For this review, take the finished solid that the model builds, in its own axes (mm). Face numbers are marked on the shaded views. A direction names the side the tool comes from. Coordinates: 2 decimals unless noted, no trailing zeros. Loops run counter-clockwise (first coordinate to the right, second up) from the corner with the lowest first, then second, coordinate; pieces in that order, holes last. Notation, with made-up numbers: M -31.5,38 L -7.5,38 A26 cw -7.5,57 Z; hole C 58.5,-35.5 d9. An arc over 180 degrees is marked long. Use one line per item in the form item = value.
```python
from build123d import *

# Parameters (mm, degrees)
SKETCH_1_W          = 45
SKETCH_1_H          = 45
EXTRUDE_1_DEPTH     = 9.8
SKETCH_2_W          = 4.7
SKETCH_2_H          = 45
EXTRUDE_2_DEPTH     = 45.7
CUT_EXTRUDE_START   = -33.6
CUT_EXTRUDE_2_DEPTH = 33.6
SKETCH_4_R          = 4
CUT_EXTRUDE_3_DEPTH = 72.630929074
SKETCH_6_R          = 6.1
CUT_EXTRUDE_5_DEPTH = 56.686533381
SKETCH_7_W          = 8.2
SKETCH_7_H          = 1
EXTRUDE_3_DEPTH     = 2
SKETCH_8_R          = 10
CUT_EXTRUDE_6_DEPTH = 4.8


# Read off the part's stored shape, not the designer's step: 切除-拉伸2
with BuildPart() as part:
    # 草图1 → 凸台-拉伸1 (new body)
    with BuildSketch(Plane.XY):
        Rectangle(SKETCH_1_W, SKETCH_1_H)
    extrude(amount=EXTRUDE_1_DEPTH)

    # 草图2 → 凸台-拉伸2 (add)
    with BuildSketch(Plane.XY.offset(9.8)):
        with Locations((-14.45, 0)):
            Rectangle(SKETCH_2_W, SKETCH_2_H)
        with Locations((14.45, 0)):
            Rectangle(SKETCH_2_W, SKETCH_2_H)
    extrude(amount=EXTRUDE_2_DEPTH)

    # 切除-拉伸2 outline → 切除-拉伸2 (cut)
    with BuildSketch(Plane.ZY.offset(16.8).offset(CUT_EXTRUDE_START)):
        with BuildLine():
            Line((55.5, 22.5), (33, 22.5))
            ThreePointArc((33, 22.5), (48.909902577, 15.909902577), (55.5, 0))
            Line((55.5, 0), (55.5, 22.5))
        make_face()
        with BuildLine():
            Line((55.5, -22.5), (55.5, 0))
            ThreePointArc((55.5, 0), (48.909902577, -15.909902577), (33, -22.5))
            Line((33, -22.5), (55.5, -22.5))
        make_face()
    extrude(amount=CUT_EXTRUDE_2_DEPTH, mode=Mode.SUBTRACT)

    # 草图4 → 切除-拉伸3 (cut, through all)
    with BuildSketch(Plane.ZY.offset(16.8)):
        with Locations((33, 0)):
            Circle(SKETCH_4_R)
    extrude(amount=-CUT_EXTRUDE_3_DEPTH, mode=Mode.SUBTRACT)

    # 草图6 → 切除-拉伸5 (cut, through all)
    with BuildSketch(Plane.XY.offset(9.8)):
        Circle(SKETCH_6_R)
    extrude(amount=-CUT_EXTRUDE_5_DEPTH, mode=Mode.SUBTRACT)

    # 草图7 → 凸台-拉伸3 (add)
    with BuildSketch(Plane(origin=(0, 0, 0), x_dir=(-1, 0, 0), z_dir=(0, 0, -1))):
        with Locations((0, 22)):
            Rectangle(SKETCH_7_W, SKETCH_7_H)
        with Locations((0, -22)):
            Rectangle(SKETCH_7_W, SKETCH_7_H)
    extrude(amount=EXTRUDE_3_DEPTH)

    # 草图8 → 切除-拉伸6 (cut)
    with BuildSketch(Plane.XY.offset(9.8)):
        Circle(SKETCH_8_R)
    extrude(amount=-CUT_EXTRUDE_6_DEPTH, mode=Mode.SUBTRACT)


solid = part.part
```
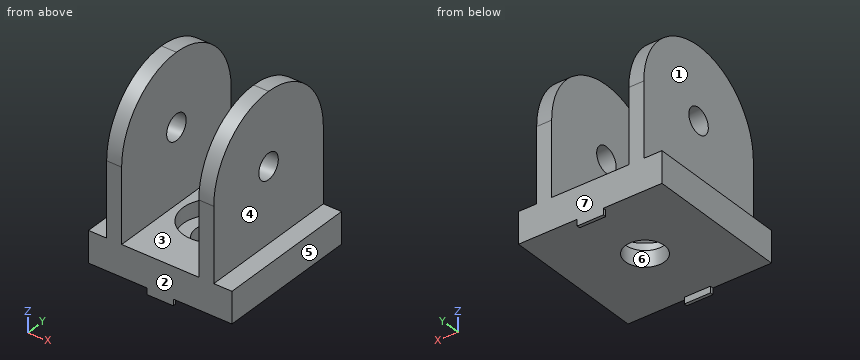
1. Draft analysis for pull direction Y (two halves, no side actions). For the marked faces 5, 6 and 7, state which applies: +Y half, -Y half, draft (parallel to the pull), parting line (faces both ways), or undercut.
Computed values:
face_5 = draft
face_6 = undercut
face_7 = +Y half
2. For pin 1 Ø3 at (x, y) = (3.5, -4.5) entering from -Z; pin 2 Ø1.1 at (y, z) = (22, -1) entering from +X; pin 3 Ø8 at (x, z) = (-15, 35) entering from +Y; pin 4 Ø12 at (y, z) = (6.5, 48.5) entering from +X, all flat-tipped, find the tip position at first contact; note any pin that passes through.
Computed values:
pin_1 = 0
pin_2 = 4.1
pin_3 = 22.5
pin_4 = 16.8
3. Consider section C-C on y = -13.5. Write out the cut boundary in (x, z), plus the area to 3 significant figures.
Computed values:
outline = M -22.5,0 L 22.5,0 L 22.5,9.8 L 16.8,9.8 L 16.8,51 L 12.1,51 L 12.1,9.8 L -12.1,9.8 L -12.1,51 L -16.8,51 L -16.8,9.8 L -22.5,9.8 Z
area = 828 mm2
4. Tool access review of the marked faces 1, 2, 3 and 4: name each direction out of +Z, -Z, +X, -X, +Y, -Y from which nothing blocks a thin tool from reaching the whole face with its end or side.
Computed values:
face_1 = +Z, -X, +Y, -Y
face_2 = +Z, -Z, +X, -X, -Y
face_3 = +Z, +Y, -Y
face_4 = +Z, +X, +Y, -Y
5. Consider section B-B on x = 0. Write out the cut boundary in (y, z).
Computed values:
outline = M -22.5,-2 L -21.5,-2 L -21.5,0 L -6.1,0 L -6.1,5 L -10,5 L -10,9.8 L -22.5,9.8 Z; M 6.1,0 L 21.5,0 L 21.5,-2 L 22.5,-2 L 22.5,9.8 L 10,9.8 L 10,5 L 6.1,5 Z
6. Wall thickness on line 1 along Y through (x, z) = (-14.9, 33); line 2 along X through (y, z) = (-13, 39); line 3 along Y through (x, z) = (0, 1.6): over which ranges is each line inside the solid? List them lowest first. Write a range as from..to.
Computed values:
line_1 = -22.5..-4, 4..22.5
line_2 = -16.8..-12.1, 12.1..16.8
line_3 = -22.5..-6.1, 6.1..22.5
7. Consider section D-D on x = 14.5. Write out the cut boundary in (y, z), plus the area to 3 significant figures.
Computed values:
outline = M -22.5,0 L 22.5,0 L 22.5,33 A22.5 ccw -22.5,33 Z; hole C 0,33 d8
area = 2,230 mm2
8. Consider section A-A on z = 23. Write out the cut boundary in (x, y), plus the area to 3 significant figures.
Computed values:
outline = M -16.8,-22.5 L -12.1,-22.5 L -12.1,22.5 L -16.8,22.5 Z; M 12.1,-22.5 L 16.8,-22.5 L 16.8,22.5 L 12.1,22.5 Z
area = 423 mm2
